Geometry: final body of the model. Coordinates: model frame, mm. A direction names the side the tool comes from. Give positions to 0.01 mm unless a question says otherwise; leave off trailing zeros. Order: outer loops, then holes, each group sorted by start corner. A loop starts at its lowest first (then second) coordinate and runs counter-clockwise, first axis right, second up. Notation, with made-up numbers: (-19.5, 59.25) -> (15.5, 59.25) arc R9 cw to (15.5, 68.25) -> close; hole circle Ø2 at (13.5, 58.5). An arc over 180 degrees is marked (long way). Write item = value, one per line.
```python
from build123d import *

# Parameters (mm, degrees)
F1_DEPTH = 25.4
F2_DEPTH = 25.4


with BuildPart() as f1:
    # F0 (on Front) → F1 (new body)
    with BuildSketch(Plane.XZ):
        Polygon((51.9276708364, 32.9955678842), (19.05, 32.9955678842), (19.05, 20.812753588), (16.2640828639, 20.812753588), (16.2640828639, 9.2959087342), (13.7671502117, 9.2959087342), (13.7671502117, 0), (51.9276708364, 0), align=None)
    extrude(amount=F1_DEPTH)

    # F0 (on Front) + F1_face (on face) → F2 (join)
    with BuildSketch(Plane.XZ):
        Polygon((19.05, 32.9955678842), (0, 0), (13.7671502117, 0), (13.7671502117, 9.2959087342), (16.2640828639, 9.2959087342), (16.2640828639, 20.812753588), (19.05, 20.812753588), align=None)
        Polygon((51.9276708364, 32.9955678842), (19.05, 32.9955678842), (19.05, 20.812753588), (16.2640828639, 20.812753588), (16.2640828639, 9.2959087342), (13.7671502117, 9.2959087342), (13.7671502117, 0), (51.9276708364, 0), align=None)
    with BuildSketch(Plane(origin=(34.1945571496, 0, 15.9589854534), x_dir=(1, 0, 0), z_dir=(0, 1, 0))):
        Polygon((-15.1445571496, -17.0365824308), (17.7331136869, -17.0365824308), (17.7331136869, 15.9589854534), (-20.4274069378, 15.9589854534), (-20.4274069378, 6.6630767192), (-17.9304742856, 6.6630767192), (-17.9304742856, -4.8537681345), (-15.1445571496, -4.8537681345), align=None)
    extrude(amount=-F2_DEPTH, dir=(0, -1, 0))


solid = f1.part
```
1) Section query C-C (y = 11). Output: boundary loops of the cut face in (x, z).
Check sheet entries:
outline = (0, 0) -> (51.93, 0) -> (51.93, 33) -> (19.05, 33) -> close
2) Section query D-D (z = 13.5). Output: boundary loops of the cut face in (x, y), plus the area to 3 significant figures.
Check sheet entries:
outline = (7.79, 0) -> (16.26, 0) -> (16.26, -25.4) -> (51.93, -25.4) -> (51.93, 25.4) -> (7.79, 25.4) -> close
area = 2,030 mm²
3) Section query A-A (y = -10.5). Output: boundary loops of the cut face in (x, z).
Check sheet entries:
outline = (13.77, 0) -> (51.93, 0) -> (51.93, 33) -> (19.05, 33) -> (19.05, 20.81) -> (16.26, 20.81) -> (16.26, 9.3) -> (13.77, 9.3) -> close
4) Reachability of faces 1 (the face through (13.767, -13, 5)), 2 (the face through (9.66, 12.52, 16.73)), 3 (the face through (19.05, -13, 27)) from +Z, -Z, +X, -X, +Y, -Y: full face, straight path, thin tool, end or side. Return the list, or none.
Check sheet entries:
face_1 = +Z, -Z, -X, -Y
face_2 = +Z, -X, +Y, -Y
face_3 = +Z, -X, -Y
5) Section query B-B (z = 7.5). Output: boundary loops of the cut face in (x, y), plus the area to 3 significant figures.
Check sheet entries:
outline = (4.33, 0) -> (13.77, 0) -> (13.77, -25.4) -> (51.93, -25.4) -> (51.93, 25.4) -> (4.33, 25.4) -> close
area = 2,180 mm²
6) Mould query, pull axis Y, two halves, no side actions, for faces 4 (the face through (33, -25.4, 17)), 5 (the face through (18, -13, 20.813)), 6 (the face through (31, 25.4, 17)). Classes: +Y half, -Y half, draft (parallel to the pull), parting line (faces both ways), or undercut.
Check sheet entries:
face_4 = -Y half
face_5 = draft
face_6 = +Y half
7) Line query: line 1 (X direction, y = -20.5, z = 10.5); line 2 (X direction, y = -3, z = 8); line 3 (Y direction, x = 9, z = 8). Output: solid intervals per line, ascending. Write a range as from..to.
Check sheet entries:
line_1 = 16.26..51.93
line_2 = 13.77..51.93
line_3 = 0..25.4
8) First-contact query: P1, Ø8, axis at x = 8.5, y = 1, coming from the +Z side; P2, Ø1, axis at y = 2.5, z = 7, coming from the -X side; P3, Ø12.5, axis at y = -7.5, z = 15, coming from the -X side. Flat tips, straight axial feed; report the tip coordinate or a pass-through.
Check sheet entries:
P1 = 21.65
P2 = 3.75
P3 = 13.77
